Source: CAD feature listing. Evaluate the final solid. Frame: model axes, mm. Face numbers are marked on the shaded views. A direction names the side the tool comes from. Coordinates: 2 decimals unless noted, no trailing zeros. Loops run counter-clockwise (first coordinate to the right, second up) from the corner with the lowest first, then second, coordinate; pieces in that order, holes last. Notation, with made-up numbers: (-9, 24) - (50, 24) arc R14 cw to (50, 43) - close; hole circle Ø9 at (-13, 41.25). An arc over 180 degrees is marked (long way). Write item = value, one per line. Start each with the question number.
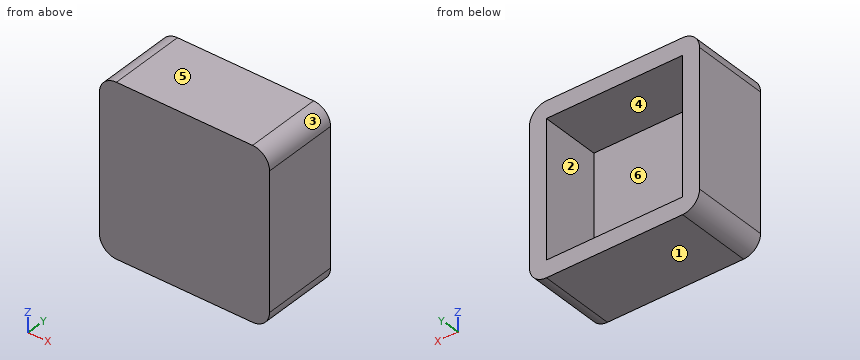
from build123d import *

# Parameters (mm, degrees)
SKETCH3_W           = 100
SKETCH3_H           = 100
BOSS_EXTRUDE1_DEPTH = 10
SKETCH4_W           = 100
SKETCH4_H           = 100
SKETCH4_W_2         = 80
SKETCH4_H_2         = 80
BOSS_EXTRUDE2_DEPTH = 35
FILLET1_R           = 10


with BuildPart() as part:
    # Sketch3 → Boss-Extrude1 (new body)
    with BuildSketch(Plane(origin=(0, 0, 0), x_dir=(1, 0, 0), z_dir=(0, 1, 0))):
        with Locations((50, 50)):
            Rectangle(SKETCH3_W, SKETCH3_H)
    extrude(amount=BOSS_EXTRUDE1_DEPTH)

    # Sketch4 → Boss-Extrude2 (add)
    with BuildSketch(Plane(origin=(0, 10, 0), x_dir=(1, 0, 0), z_dir=(0, 1, 0))):
        with Locations((50, 50)):
            Rectangle(SKETCH4_W, SKETCH4_H)
        with Locations((50, 50)):
            Rectangle(SKETCH4_W_2, SKETCH4_H_2, mode=Mode.SUBTRACT)
    extrude(amount=BOSS_EXTRUDE2_DEPTH)

    # Fillet1
    fillet1_edges = [part.edges().sort_by_distance(p)[0] for p in [
        (0, 22.5, -100),
        (100, 22.5, -100),
        (100, 22.5, 0),
        (0, 22.5, 0),
    ]]
    fillet(fillet1_edges, radius=FILLET1_R)


solid = part.part
Item 1: Reachability of the marked faces 1 and 2 from +Z, -Z, +X, -X, +Y, -Y: full face, straight path, thin tool, end or side. Return the list, or none.
Item 2: Cut plane B-B (y = 28.5). Return the cut outline in (x, z), then the cut area to 3 significant figures.
Item 3: First-contact query: pin 1 (1.5 mm diameter, centred on x = 80, z = -53, fed in from +Y). Flat tip, straight axial feed; report the tip coordinate or a pass-through.
Item 4: Cut plane D-D (x = 94). Return the cut outline in (y, z).
Item 5: Cut plane C-C (x = 35.5). Return the cut outline in (y, z).
Item 6: Cut plane A-A (z = -64). Return the cut outline in (x, y).
Item 7: Material intervals for L1, parallel to Z at x = 14, y = 34; L2, parallel to X at y = 13.5, z = -16.5; L3, parallel to Y at x = 17, z = -46, sorted ascending. Write a range as [from, to].
Item 8: Draft query along X for the marked faces 3, 4, 5 and 6. Return one class per face: released by +X, released by -X, zero draft, split by the parting line, or undercut.
Responses:
q1.face_1 = -Z, +X, -X, +Y, -Y
q1.face_2 = +Y
q2.outline = (0, -90) arc R10 ccw to (10, -100) - (90, -100) arc R10 ccw to (100, -90) - (100, -10) arc R10 ccw to (90, 0) - (10, 0) arc R10 ccw to (0, -10) - close; hole (10, -90) - (90, -90) - (90, -10) - (10, -10) - close
q2.area = 3,510 mm2
q3.pin_1 = 10
q4.outline = (0, -99.17) - (45, -99.17) - (45, -0.83) - (0, -0.83) - close
q5.outline = (0, -100) - (45, -100) - (45, -90) - (10, -90) - (10, -10) - (45, -10) - (45, 0) - (0, 0) - close
q6.outline = (0, 0) - (100, 0) - (100, 45) - (90, 45) - (90, 10) - (10, 10) - (10, 45) - (0, 45) - close
q7.L1 = [-100, -90], [-10, 0]
q7.L2 = [0, 10], [90, 100]
q7.L3 = [0, 10]
q8.face_3 = released by +X
q8.face_4 = undercut
q8.face_5 = zero draft
q8.face_6 = undercut
